```python
from build123d import *

# Parameters (mm, degrees)
SKETCH1_R                               = 4
BOSS_EXTRUDE1_DEPTH                     = 100
CBORE_FOR_M5_HEX_HEAD_BOLT2_D           = 13.5
CBORE_FOR_M5_HEX_HEAD_BOLT2_DEPTH       = 23.85
CBORE_FOR_M5_HEX_HEAD_BOLT2_CBORE_D     = 32
CBORE_FOR_M5_HEX_HEAD_BOLT2_CBORE_DEPTH = 5
CBORE_FOR_M5_HEX_HEAD_BOLT3_D           = 10.2
CBORE_FOR_M5_HEX_HEAD_BOLT3_DEPTH       = 13.5
CBORE_FOR_M5_HEX_HEAD_BOLT3_CBORE_D     = 22
CBORE_FOR_M5_HEX_HEAD_BOLT3_CBORE_DEPTH = 3.5


with BuildPart() as part:
    # Sketch1 → Boss-Extrude1 (new body)
    with BuildSketch(Plane(origin=(0, 0, 0), x_dir=(1, 0, 0), z_dir=(0, 1, 0))):
        Polygon((-32.5, 0), (0, 0), (0, 25), (32, 25), (32, -40), (-32.5, -40), align=None)
        with Locations(Location((-12.5, -20, 0), (0, 0, 90))):
            Circle(SKETCH1_R, mode=Mode.SUBTRACT)
        with Locations(Location((16, 12.5, 0), (0, 0, 90))):
            Circle(SKETCH1_R, mode=Mode.SUBTRACT)
    extrude(amount=BOSS_EXTRUDE1_DEPTH)

    # CBORE for M5 Hex Head Bolt2
    with Locations(Plane(origin=(0, 0, 0), x_dir=(-1, 0, 0), z_dir=(0, -1, 0))):
        with Locations((12.5, -20)):
            CounterBoreHole(CBORE_FOR_M5_HEX_HEAD_BOLT2_D / 2, CBORE_FOR_M5_HEX_HEAD_BOLT2_CBORE_D / 2, CBORE_FOR_M5_HEX_HEAD_BOLT2_CBORE_DEPTH, depth=CBORE_FOR_M5_HEX_HEAD_BOLT2_DEPTH)

    # CBORE for M5 Hex Head Bolt3
    with Locations(Plane(origin=(0, 0, 0), x_dir=(-1, 0, 0), z_dir=(0, -1, 0))):
        with Locations((-16, 12.5)):
            CounterBoreHole(CBORE_FOR_M5_HEX_HEAD_BOLT3_D / 2, CBORE_FOR_M5_HEX_HEAD_BOLT3_CBORE_D / 2, CBORE_FOR_M5_HEX_HEAD_BOLT3_CBORE_DEPTH, depth=CBORE_FOR_M5_HEX_HEAD_BOLT3_DEPTH)


solid = part.part
```
Verification items for the finished model (mm, model axes). A direction names the side the tool comes from. Round coordinates to 2 decimals unless told otherwise and drop trailing zeros. Write each loop counter-clockwise with the first axis right and the second up, starting at its lowest first coordinate (ties: lowest second). Pieces come first, ordered by that corner, then holes. Notation, with made-up numbers: (2.25, -16) - (61.25, -16) arc R28 cw to (61.25, 20) - close; hole circle Ø8 at (41, -12). An arc over 180 degrees is marked (long way). Answer as a JSON object with one key per item and string values. Group by question number.
Q1. Mould release check, pull along Z, two halves, no side actions. Record for faces 4 (the flat face through (0, 49, 40)), 5 (the cylindrical face through (-6.062, 14.557, 17.972)), 6 (the flat face through (7, 0, 14)): released by +Z, released by -Z, zero draft, split by the parting line, or undercut.
Q2. Go/stop test with flat-tipped pins: pin 1 Ø3 at (y, z) = (52.5, -8.5) entering from -X; pin 2 Ø16 at (x, y) = (-18.5, 70.5) entering from -Z; pin 3 Ø8 at (x, z) = (16, -12) entering from -Y. Record where each tip stops, or that it passes through.
Q3. Thickness scan on line 1 (Z direction, x = 16, y = 59); line 2 (X direction, y = 2, z = -12); line 3 (Z direction, x = -4.5, y = 78.5). Record the ranges inside material, lowest first.
Q4. Section check C-C, the plane y = 71.5. Enter the section's corners in (x, z).
Q5. Section check D-D, the plane x = -3. Enter the section's corners in (y, z).
Q6. Section check A-A, the plane z = -12.5. Enter the section's corners in (x, y), plus the area to 3 significant figures.
Q7. Section check B-B, the plane x = 16. Enter the section's corners in (y, z), plus the area to 3 significant figures.
Q8. Tool access check on faces 1 (the flat face through (12, 13.5, -11)), 2 (the flat face through (-16, 49, 0)), 3 (the flat face through (16, 49, -25)). Record the directions out of +Z, -Z, +X, -X, +Y, -Y that give a thin tool (end or side, any length) a straight path to the whole face; none if there is none.
Found:
{
 "1": {"face 4": "released by +Z", "face 5": "undercut", "face 6": "zero draft"},
 "2": {"pin 1": "stops at x = 0", "pin 2": "stops at z = 0", "pin 3": "stops at y = 13.5"},
 "3": {"line 1": "z = -25 to -16.5, -8.5 to 40", "line 2": "x = 0 to 5.01, 26.99 to 32", "line 3": "z = 0 to 40"},
 "4": {"outline": "(-32.5, 0) - (0, 0) - (0, -25) - (32, -25) - (32, 40) - (-32.5, 40) - close; hole circle Ø8 at (-12.5, 20); hole circle Ø8 at (16, -12.5)"},
 "5": {"outline": "(0, 0) - (100, 0) - (100, 40) - (0, 40) - (0, 32.87) - (5, 32.87) - (5, 7.13) - (0, 7.13) - close"},
 "6": {"outline": "(0, 0) - (5, 0) - (5, 3.5) - (10.9, 3.5) - (10.9, 13.5) - (12, 13.5) - (12, 100) - (0, 100) - close; (20, 13.5) - (21.1, 13.5) - (21.1, 3.5) - (27, 3.5) - (27, 0) - (32, 0) - (32, 100) - (20, 100) - close", "area": "2,330 mm^2"},
 "7": {"outline": "(0, -25) - (100, -25) - (100, -16.5) - (13.5, -16.5) - (13.5, -17.6) - (3.5, -17.6) - (3.5, -23.5) - (0, -23.5) - close; (0, -1.5) - (3.5, -1.5) - (3.5, -7.4) - (13.5, -7.4) - (13.5, -8.5) - (100, -8.5) - (100, 40) - (0, 40) - close", "area": "5,630 mm^2"},
 "8": {"face 1": "-Y", "face 2": "-Z, -X, +Y, -Y", "face 3": "-Z, +X, -X, +Y, -Y"}
}
